For this review, take the finished solid that the model builds, in its own axes (mm). Give positions to 0.01 mm unless a question says otherwise; leave off trailing zeros. Order: outer loops, then holes, each group sorted by start corner. A loop starts at its lowest first (then second) coordinate and runs counter-clockwise, first axis right, second up. Notation, with made-up numbers: (23.5, 84.25) - (80.5, 84.25) arc R28 ccw to (80.5, 118.25) - close; hole circle Ø4 at (78.5, 87). An arc over 180 degrees is marked (long way). Put each result on its own line as item: value. Start each with the question number.
```python
from build123d import *

# Parameters (mm, degrees)
SKETCH1_R                            = 4.7625
BOSS_EXTRUDE1_DEPTH                  = 50.8
F_10_32_TAPPED_HOLE1_D               = 4.0386
F_10_32_TAPPED_HOLE1_DEPTH           = 11.938
F_10_32_TAPPED_HOLE1_TIP             = 1.213317848
F_10_32_TAPPED_HOLE1_ON_FACE_2_D     = 4.0386
F_10_32_TAPPED_HOLE1_ON_FACE_2_DEPTH = 11.938
F_10_32_TAPPED_HOLE1_ON_FACE_2_TIP   = 1.213317848


with BuildPart() as part:
    # Sketch1 → Boss-Extrude1 (new body, symmetric)
    with BuildSketch(Plane(origin=(0, 0, 0), x_dir=(1, 0, 0), z_dir=(0, 1, 0))):
        Circle(SKETCH1_R)
    extrude(amount=BOSS_EXTRUDE1_DEPTH, both=True)

    # #10-32 Tapped Hole1
    with Locations(Plane.ZX.offset(50.8)):
        with Locations((0, 0)):
            Hole(F_10_32_TAPPED_HOLE1_D / 2, depth=F_10_32_TAPPED_HOLE1_DEPTH)
            with Locations((0, 0, -(F_10_32_TAPPED_HOLE1_DEPTH + F_10_32_TAPPED_HOLE1_TIP / 2))):  # 118° drill point
                Cone(0, F_10_32_TAPPED_HOLE1_D / 2, F_10_32_TAPPED_HOLE1_TIP, mode=Mode.SUBTRACT)

    # #10-32 Tapped Hole1 on face 2
    with Locations(Plane(origin=(0, -50.8, 0), x_dir=(0, 0, -1), z_dir=(0, -1, 0))):
        with Locations((0, 0)):
            Hole(F_10_32_TAPPED_HOLE1_ON_FACE_2_D / 2, depth=F_10_32_TAPPED_HOLE1_ON_FACE_2_DEPTH)
            with Locations((0, 0, -(F_10_32_TAPPED_HOLE1_ON_FACE_2_DEPTH + F_10_32_TAPPED_HOLE1_ON_FACE_2_TIP / 2))):  # 118° drill point
                Cone(0, F_10_32_TAPPED_HOLE1_ON_FACE_2_D / 2, F_10_32_TAPPED_HOLE1_ON_FACE_2_TIP, mode=Mode.SUBTRACT)


solid = part.part
```
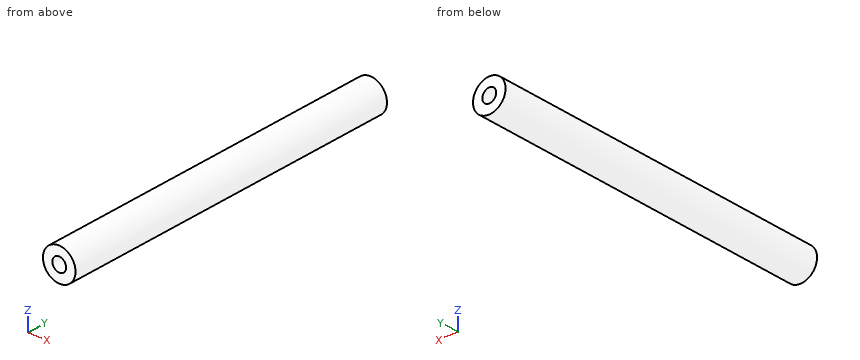
1. Wall thickness on line 1 (X direction, y = 45.75, z = 0); line 2 (X direction, y = -8, z = -3): over which ranges is each line inside the solid? List them lowest first. Write a range as from..to.
2. Add section C-C, the plane x = -3.75. Give the boundary of the cut face in (y, z).
3. Add section B-B, the plane z = 3. Give the boundary of the cut face in (x, y).
4. Add section A-A, the plane y = 23. Give the boundary of the cut face in (x, z) (1 decimal), then the cut area to 3 significant figures.
5. Clearance check with flat-ended pins moving along their axes: pin 1 (1 mm diameter, centred on x = -2.5, y = -20, fed in from -Z); pin 2 (3 mm diameter, centred on x = -1.5, y = -15, fed in from -Z); pin 3 (4 mm diameter, centred on x = -3, y = 18, fed in from -Z). State where each tip first meets the part, or that it passes through.
Found:
1. line 1: x = -4.76..-2.02, 2.02..4.76
1. line 2: x = -3.7..3.7
2. outline: (-50.8, -2.94) - (50.8, -2.94) - (50.8, 2.94) - (-50.8, 2.94) - close
3. outline: (-3.7, -50.8) - (3.7, -50.8) - (3.7, 50.8) - (-3.7, 50.8) - close
4. outline: circle Ø9.5 at (0, 0)
4. area: 71.3 mm^2
5. pin 1: stops at z = -4.32
5. pin 2: stops at z = -4.76
5. pin 3: stops at z = -4.66
